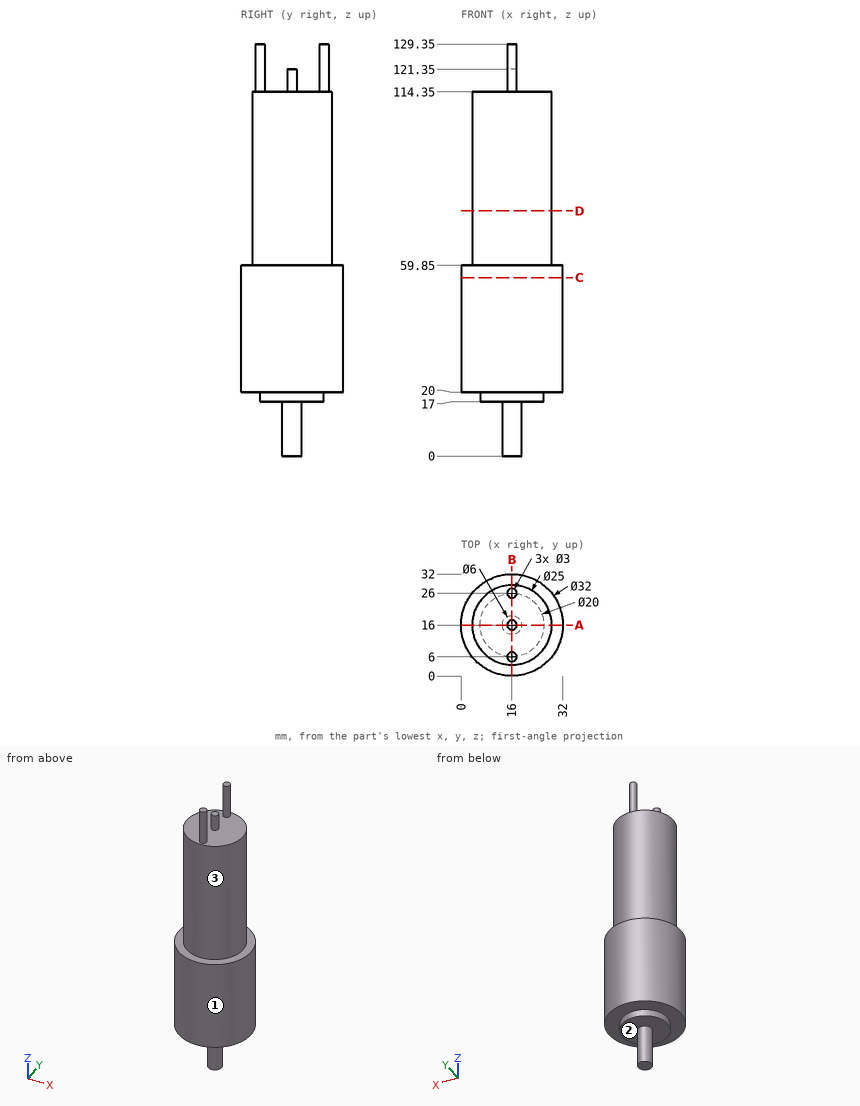
Study the drawing (mm; zero at the part's minimum x, y, z) and answer. A direction names the side the tool comes from. Give positions to 0.01 mm unless a question says otherwise; leave off trailing zeros. Write each loop counter-clockwise with the first axis right and the second up, starting at its lowest first coordinate (ties: lowest second). Pieces come first, ordered by that corner, then holes. Notation, with made-up numbers: (-8.75, -33.75) -> (46.25, -33.75) arc R30 ccw to (46.25, 0.25) -> close; hole circle Ø8 at (4.25, -25.5). An arc over 180 degrees is marked (long way). Answer as a JSON object with one key per item and string values. Group by question number.
1) A tool of negligible diameter and unlimited length cuts with its end or side. For the marked faces 1, 2 and 3, from which of +Z, -Z, +X, -X, +Y, -Y can it reach the whole face along a straight path? Write none if from no direction.
2) Find section A-A (y = 16). Write down the section's boundary in (x, z).
3) Find section D-D (z = 77). Write down the section's boundary in (x, y), and give its area (3 significant figures).
4) Consider L1, parallel to Z at x = 18.5, y = 4.5; L2, parallel to Z at x = 18.5, y = 29; L3, parallel to Y at x = 3.5, z = 49.5. Determine where each line is inside the solid, lowest interval first. Write a range as from..to.
5) Find section C-C (z = 56). Write down the section's boundary in (x, y), and give its area (3 significant figures).
6) Find section B-B (x = 16). Write down the section's boundary in (y, z), and give its area (3 significant figures).
7) Each of these flat-tipped pins is pushed along its axis until it touches: P1, Ø3, axis at x = 12.5, z = 61, coming from the +Y side; P2, Ø5, axis at y = 11.5, z = 79.5, coming from the -X side; P3, Ø10, axis at x = 20, y = 7.5, coming from the -Z side; P4, Ø8, axis at x = 15.5, z = 63.5, coming from the -Y side. Where does it stop, or does it pass through?
Values follow:
{
 "1": {"face 1": "+Z, -Z", "face 2": "-Z", "face 3": "+Z"},
 "2": {"outline": "(0, 20) -> (6, 20) -> (6, 17) -> (13, 17) -> (13, 0) -> (19, 0) -> (19, 17) -> (26, 17) -> (26, 20) -> (32, 20) -> (32, 59.85) -> (28.5, 59.85) -> (28.5, 114.35) -> (17.5, 114.35) -> (17.5, 121.35) -> (14.5, 121.35) -> (14.5, 114.35) -> (3.5, 114.35) -> (3.5, 59.85) -> (0, 59.85) -> close"},
 "3": {"outline": "circle Ø25 at (16, 16)", "area": "491 mm2"},
 "4": {"L1": "z = 20..114.35", "L2": "z = 20..59.85", "L3": "y = 6.01..25.99"},
 "5": {"outline": "circle Ø32 at (16, 16)", "area": "804 mm2"},
 "6": {"outline": "(0, 20) -> (6, 20) -> (6, 17) -> (13, 17) -> (13, 0) -> (19, 0) -> (19, 17) -> (26, 17) -> (26, 20) -> (32, 20) -> (32, 59.85) -> (28.5, 59.85) -> (28.5, 114.35) -> (27.5, 114.35) -> (27.5, 129.35) -> (24.5, 129.35) -> (24.5, 114.35) -> (17.5, 114.35) -> (17.5, 121.35) -> (14.5, 121.35) -> (14.5, 114.35) -> (7.5, 114.35) -> (7.5, 129.35) -> (4.5, 129.35) -> (4.5, 114.35) -> (3.5, 114.35) -> (3.5, 59.85) -> (0, 59.85) -> close", "area": "2,910 mm2"},
 "7": {"P1": "stops at y = 31.8", "P2": "stops at x = 3.66", "P3": "stops at z = 17", "P4": "stops at y = 0"}
}
